Geometry check sheet. Reference: the model listing, model coordinates, mm. A direction names the side the tool comes from. Round coordinates to 2 decimals unless told otherwise and drop trailing zeros. Loops run counter-clockwise (first coordinate to the right, second up) from the corner with the lowest first, then second, coordinate; pieces in that order, holes last. Notation, with made-up numbers: (75, 0) -> (116, 0) arc R22 ccw to (116, 6) -> close; hole circle Ø7 at (7, 55). An arc over 180 degrees is marked (long way). Use one line per item in the form item = value.
from build123d import *

# Parameters (mm, degrees)
F2_DEPTH = 16.75
F4_DEPTH = 16.001
F5_R     = 3.429
F6_R     = 3.429
F7_DEPTH = 3
F8_R     = 5
F9_R     = 5
F10_R    = 5
F11_R    = 5


with BuildPart() as f2:
    # F1 (on Front) → F2 (new body, symmetric)
    with BuildSketch(Plane.XZ):
        Polygon((-84.0640169114, 3), (-84.0640169114, 0), (-63.7959806109, 0), (-18.5640169114, 13), (11.4359830886, 13), (56.667946788, 0), (76.9359830886, 0), (76.9359830886, 3), (57.0905048336, 3), (11.8585411342, 16), (-18.986574957, 16), (-64.2185386565, 3), align=None)
    extrude(amount=F2_DEPTH, both=True)

    # F3 (on face) → F4 (cut, through all)
    with BuildSketch(Plane.XY.offset(16)):
        with BuildLine():
            ThreePointArc((-3.5640168758, -14.25), (6.5122547331, -10.0762716193), (10.6859830886, 0))
            ThreePointArc((10.6859830886, 0), (6.5122547205, 10.0762716319), (-3.5640169114, 14.25))
            ThreePointArc((-3.5640169114, 14.25), (-17.8140169114, -1.78e-08), (-3.5640168758, -14.25))
        make_face()
    extrude(amount=-F4_DEPTH, mode=Mode.SUBTRACT)

    # F5 (on face) + F6 (on face) → F7 (join)
    with BuildSketch(Plane(origin=(0, 0, 0), x_dir=(1, 0, 0), z_dir=(0, 0, -1))):
        with Locations((-79.0640169114, 0)):
            Circle(F5_R)
    with BuildSketch(Plane(origin=(0, 0, 0), x_dir=(1, 0, 0), z_dir=(0, 0, -1))):
        with Locations((71.9359830886, 0)):
            Circle(F6_R)
    extrude(amount=F7_DEPTH)

    # F8
    f8_edges = [f2.edges().sort_by_distance(p)[0] for p in [
        (-84.064017, -16.75, 1.5),
    ]]
    fillet(f8_edges, radius=F8_R)

    # F9
    f9_edges = [f2.edges().sort_by_distance(p)[0] for p in [
        (-84.064017, 16.75, 1.5),
    ]]
    fillet(f9_edges, radius=F9_R)

    # F10
    f10_edges = [f2.edges().sort_by_distance(p)[0] for p in [
        (76.935983, -16.75, 1.5),
    ]]
    fillet(f10_edges, radius=F10_R)

    # F11
    f11_edges = [f2.edges().sort_by_distance(p)[0] for p in [
        (76.935983, 16.75, 1.5),
    ]]
    fillet(f11_edges, radius=F11_R)


solid = f2.part
1. Material ranges on line 1 along Z through (x, y) = (69, -14); line 2 along Z through (x, y) = (-15.5, 11.5); line 3 along X through (y, z) = (-3, -1.5), recorded low to high.
Return value:
line_1 = 0 to 3
line_2 = 13 to 16
line_3 = -80.72 to -77.4, 70.28 to 73.6
2. Tool access check on faces 4 (the cylindrical face through (-75.896, 1.313, -1.479)), 5 (the flat face through (-41.5, -0.23, 6.41)), 6 (the flat face through (76.936, 0, 1)), 7 (the flat face through (67, 0, 3)). Record the directions out of +Z, -Z, +X, -X, +Y, -Y that give a thin tool (end or side, any length) a straight path to the whole face; none if there is none.
Return value:
face_4 = -Z
face_5 = -Z, +Y, -Y
face_6 = +Z, -Z, +X, +Y, -Y
face_7 = +Z, +X, +Y, -Y
3. Section check A-A (z = 10.5). Record the boundary of the cut face in (x, y).
Return value:
outline = (-38.12, -16.75) -> (-27.26, -16.75) -> (-27.26, 16.75) -> (-38.12, 16.75) -> close; (20.13, -16.75) -> (31, -16.75) -> (31, 16.75) -> (20.13, 16.75) -> close
4. Mould release check, pull along X, two halves, no side actions. Record for faces 1 (the flat face through (-74, 0, 3)), 2 (the cylindrical face through (-82.638, 15.246, 1.479)), 3 (the flat face through (33.7, -0.2, 6.6)): released by +X, released by -X, zero draft, split by the parting line, or undercut.
Return value:
face_1 = zero draft
face_2 = released by -X
face_3 = undercut
5. Section check B-B (y = 6.5). Record the boundary of the cut face in (x, z), then the cut area to 3 significant figures.
Return value:
outline = (-84.06, 0) -> (-63.8, 0) -> (-18.56, 13) -> (-16.25, 13) -> (-16.25, 16) -> (-18.99, 16) -> (-64.22, 3) -> (-84.06, 3) -> close; (9.12, 13) -> (11.44, 13) -> (56.67, 0) -> (76.94, 0) -> (76.94, 3) -> (57.09, 3) -> (11.86, 16) -> (9.12, 16) -> close
area = 418 mm2
6. Section check C-C (x = 14). Record the boundary of the cut face in (y, z).
Return value:
outline = (-16.75, 12.26) -> (16.75, 12.26) -> (16.75, 15.38) -> (-16.75, 15.38) -> close
7. Gauge pin test, flat ends, axial feed: pin 1 (10 mm diameter, centred on x = -79, y = -0.5, fed in from +Z); pin 2 (1 mm diameter, centred on x = -31, y = 9.5, fed in from -Z); pin 3 (10 mm diameter, centred on x = -36.5, y = -1, fed in from +Z). Record the tip position at first contact, or that the pin passes through.
Return value:
pin_1 = 3
pin_2 = 9.28
pin_3 = 12.4
